Geometry: final body of the model. Coordinates: model frame, mm. A direction names the side the tool comes from. Give positions to 0.01 mm unless a question says otherwise; leave off trailing zeros. Order: outer loops, then holes, each group sorted by start corner. A loop starts at its lowest first (then second) coordinate and runs counter-clockwise, first axis right, second up. Notation, with made-up numbers: (46.5, 14.5) -> (56.5, 14.5) arc R23 ccw to (56.5, 51.5) -> close; hole circle Ø4 at (27, 34). An arc over 180 degrees is marked (long way). Answer in a Markdown table with one row per item. Add a question column.
Q1. Cut plane D-D on z = 12. Return the cut outline in (x, y).
Q2. Cut plane C-C on y = -73. Return the cut outline in (x, z), and give its area (3 significant figures).
Q3. Set-up query: faces 1 (the face through (-8.2, -2.54, 24.2)), 2 (the face through (10.583, -63, 0)), 3 (the face through (0, -63, 5.001)), 4 (the face through (0, -63, -5.001)). Return all of +Z, -Z, +X, -X, +Y, -Y with unobstructed straight access to the full face (end or side cutting, diameter ignored); none if empty.
Q4. Cut plane B-B on z = 0. Return the cut outline in (x, y), and give its area (3 significant figures).
Q5. Contact query for flat-ended pins moving along their axis: P1, Ø5, axis at y = -59, z = -1, coming from the -X side; P2, Ø17, axis at x = 2.5, y = -51, coming from the +Z side; P3, Ø12, axis at x = 7.5, y = -65.5, coming from the -Z side; P4, Ø6, axis at y = -91, z = -11, coming from the -X side. Output: stop coordinate, or through.
Q6. Line query: line 1 along Y through (x, z) = (-14, 17); line 2 along X through (y, z) = (-79, -1); line 3 along Z through (x, y) = (9, -83). Output: solid intervals per line, ascending. Write a range as from..to.
Q7. Cut plane A-A on x = 0. Return the cut outline in (y, z).
from build123d import *

# Parameters (mm, degrees)
F0_R     = 25.4
F1_DEPTH = 25.4
F2_W     = 21.16544
F2_H     = 10.00125
F3_DEPTH = 101.6
F4_R     = 27.102651
F5_DEPTH = 2.54


with BuildPart() as f1:
    # F0 (on Front) → F1 (new body)
    with BuildSketch(Plane.XZ):
        Circle(F0_R)
    extrude(amount=F1_DEPTH)

    # F2 (on Front) → F3 (join)
    with BuildSketch(Plane.XZ):
        Rectangle(F2_W, F2_H)
    extrude(amount=F3_DEPTH)

    # F4 (on Front) → F5 (join)
    with BuildSketch(Plane.XZ):
        Circle(F4_R)
    extrude(amount=F5_DEPTH)


solid = f1.part
Completed:
| question | item | result |
|---|---|---|
| 1 | outline | (-24.3, -2.54) -> (-22.39, -2.54) -> (-22.39, -25.4) -> (22.39, -25.4) -> (22.39, -2.54) -> (24.3, -2.54) -> (24.3, 0) -> (-24.3, 0) -> close |
| 2 | outline | (-10.58, -5) -> (10.58, -5) -> (10.58, 5) -> (-10.58, 5) -> close |
| 2 | area | 212 mm² |
| 3 | face 1 | -Y |
| 3 | face 2 | +Z, -Z, +X, -Y |
| 3 | face 3 | +Z, +X, -X, -Y |
| 3 | face 4 | -Z, +X, -X, -Y |
| 4 | outline | (-27.1, -2.54) -> (-25.4, -2.54) -> (-25.4, -25.4) -> (-10.58, -25.4) -> (-10.58, -101.6) -> (10.58, -101.6) -> (10.58, -25.4) -> (25.4, -25.4) -> (25.4, -2.54) -> (27.1, -2.54) -> (27.1, 0) -> (-27.1, 0) -> close |
| 4 | area | 2,910 mm² |
| 5 | P1 | stops at x = -10.58 |
| 5 | P2 | stops at z = 5 |
| 5 | P3 | stops at z = -5 |
| 5 | P4 | passes through |
| 6 | line 1 | y = -25.4..0 |
| 6 | line 2 | x = -10.58..10.58 |
| 6 | line 3 | z = -5..5 |
| 7 | outline | (-101.6, -5) -> (-25.4, -5) -> (-25.4, -25.4) -> (-2.54, -25.4) -> (-2.54, -27.1) -> (0, -27.1) -> (0, 27.1) -> (-2.54, 27.1) -> (-2.54, 25.4) -> (-25.4, 25.4) -> (-25.4, 5) -> (-101.6, 5) -> close |
